from build123d import *

# Parameters (mm, degrees)
F0_R     = 1.5
F0_W     = 3.175
F0_H     = 19.05
F0_W_2   = 10.5
F0_H_2   = 27
F1_DEPTH = 12.7


with BuildPart() as f1:
    # F0 (on Front) → F1 (new body)
    with BuildSketch(Plane.XZ):
        Polygon((-85.725, 161.925), (-161.925, 161.925), (-161.925, 85.725), (-146.685, 72.43161), (-146.685, -72.43161), (-161.925, -85.725), (-161.925, -161.925), (-85.725, -161.925), (-72.43161, -146.685), (72.43161, -146.685), (85.725, -161.925), (161.925, -161.925), (161.925, -85.725), (146.685, -72.43161), (146.685, 72.43161), (161.925, 85.725), (161.925, 161.925), (85.725, 161.925), (72.43161, 146.685), (63.7538, 146.685), (63.7538, -5.715), (-5.2462, -5.715), (-5.2462, 146.685), (-72.43161, 146.685), align=None)
        with Locations((-146.925, -156.925)):
            Circle(F0_R, mode=Mode.SUBTRACT)
        with Locations((-156.925, -146.925)):
            Circle(F0_R, mode=Mode.SUBTRACT)
        with Locations((-153.9875, -123.825)):
            Rectangle(F0_W, F0_H, mode=Mode.SUBTRACT)
        with Locations((-94.9964, -72.225)):
            Circle(F0_R, mode=Mode.SUBTRACT)
        with Locations((-84.9962, -72.225)):
            Rectangle(F0_W_2, F0_H_2, mode=Mode.SUBTRACT)
        with Locations((-74.9964, -72.225)):
            Circle(F0_R, mode=Mode.SUBTRACT)
        with Locations((146.925, -156.925)):
            Circle(F0_R, mode=Mode.SUBTRACT)
        with Locations((156.925, -146.925)):
            Circle(F0_R, mode=Mode.SUBTRACT)
        with Locations((153.9875, -123.825)):
            Rectangle(F0_W, F0_H, mode=Mode.SUBTRACT)
        with Locations((75.0036, -72.225)):
            Circle(F0_R, mode=Mode.SUBTRACT)
        with Locations((85.0038, -72.225)):
            Rectangle(F0_W_2, F0_H_2, mode=Mode.SUBTRACT)
        with Locations((95.0036, -72.225)):
            Circle(F0_R, mode=Mode.SUBTRACT)
        with Locations((-94.9964, 72.225)):
            Circle(F0_R, mode=Mode.SUBTRACT)
        with Locations((-84.9962, 72.225)):
            Rectangle(F0_W_2, F0_H_2, mode=Mode.SUBTRACT)
        with Locations((-74.9964, 72.225)):
            Circle(F0_R, mode=Mode.SUBTRACT)
        with Locations((-153.9875, 123.825)):
            Rectangle(F0_W, F0_H, mode=Mode.SUBTRACT)
        with Locations((-156.925, 146.925)):
            Circle(F0_R, mode=Mode.SUBTRACT)
        with Locations((-146.925, 156.925)):
            Circle(F0_R, mode=Mode.SUBTRACT)
        with Locations((75.0036, 72.225)):
            Circle(F0_R, mode=Mode.SUBTRACT)
        with Locations((85.0038, 72.225)):
            Rectangle(F0_W_2, F0_H_2, mode=Mode.SUBTRACT)
        with Locations((95.0036, 72.225)):
            Circle(F0_R, mode=Mode.SUBTRACT)
        with Locations((153.9875, 123.825)):
            Rectangle(F0_W, F0_H, mode=Mode.SUBTRACT)
        with Locations((156.925, 146.925)):
            Circle(F0_R, mode=Mode.SUBTRACT)
        with Locations((146.925, 156.925)):
            Circle(F0_R, mode=Mode.SUBTRACT)
        Polygon((-146.685, 72.43161), (-161.925, 85.725), (-161.925, -85.725), (-146.685, -72.43161), align=None)
    extrude(amount=F1_DEPTH)


solid = f1.part
Read the model definition and answer for the solid it produces. Units are mm, in the model's axes. A direction names the side the tool comes from. Coordinates: 2 decimals unless noted, no trailing zeros. Loops run counter-clockwise (first coordinate to the right, second up) from the corner with the lowest first, then second, coordinate; pieces in that order, holes last. Notation, with made-up numbers: (-8, 48.25) - (51, 48.25) arc R16 ccw to (51, 70.25) - close; hole circle Ø5 at (26.5, -4.5). An arc over 180 degrees is marked (long way). Answer in a Markdown table with one row per item.
Q1. Straight lines are drawn through the part: line 1 along X through (y, z) = (-8.5, -119) (3 decimals); line 2 along X through (y, z) = (-8.75, -85.5) (3 decimals); line 3 along X through (y, z) = (-3.5, 89) (3 decimals). For each, find the intervals that lie inside material, in ascending order. Write a range as [from, to].
Here are the results:
| item | result |
|---|---|
| line 1 | x = [-161.925, -155.575], [-152.4, 152.4], [155.575, 161.925] |
| line 2 | x = [-161.925, -90.246], [-79.746, 79.754], [90.254, 161.667] |
| line 3 | x = [-161.925, -5.246], [63.754, 161.925] |
Q2. Find section B-B on z = 43. Write down the section's boundary in (x, y) (3 decimals).
Here are the results:
| item | result |
|---|---|
| outline | (-161.925, -12.7) - (-5.246, -12.7) - (-5.246, 0) - (-161.925, 0) - close; (63.754, -12.7) - (146.685, -12.7) - (146.685, 0) - (63.754, 0) - close |
Q3. The mould has two halves that part along X. Classify faces 1 (the flat face through (-161.925, -6, 2)), 2 (the flat face through (79.17, -6.26, 154.41)), 3 (the flat face through (-123, -6, 161.925)), 4 (the flat face through (154.198, -6.261, 78.985)): pulls with the +X half, pulls with the -X half, needs draft (parallel to the pull), parting line crosses it, or undercut.
Here are the results:
| item | result |
|---|---|
| face 1 | pulls with the -X half |
| face 2 | undercut |
| face 3 | needs draft |
| face 4 | pulls with the +X half |
Q4. For faces 5 (the flat face through (154.41, -6.26, -79.17)), 6 (the flat face through (161.925, -6, -124)), 7 (the flat face through (90.254, -6, -72)), 8 (the flat face through (68, -6, 146.685)), 9 (the flat face through (-1, -6, -146.685)), determine the directions among +Z, -Z, +X, -X, +Y, -Y from which every point of the face is accessible in a straight line to the end or side of a thin tool.
Here are the results:
| item | result |
|---|---|
| face 5 | +X, +Y, -Y |
| face 6 | +Z, -Z, +X, +Y, -Y |
| face 7 | +Y, -Y |
| face 8 | +Z, +Y, -Y |
| face 9 | -Z, +Y, -Y |
Q5. Given P1, Ø4, axis at x = -3, y = -9, coming from the -Z side (3 decimals); P2, Ø6, axis at x = -1, z = 112, coming from the -Y side; P3, Ø5, axis at x = -84, y = -6, coming from the -Z side (3 decimals); P4, Ø4, axis at y = -7.5, z = -67.5, coming from the +X side (3 decimals), each flat-ended and moving along its own axis, determine where each tip first touches the part or whether it passes through.
Here are the results:
| item | result |
|---|---|
| P1 | stops at z = -146.685 |
| P2 | passes through |
| P3 | stops at z = -161.925 |
| P4 | stops at x = 146.685 |
Q6. Find section A-A on z = 120. Write down the section's boundary in (x, y) (3 decimals).
Here are the results:
| item | result |
|---|---|
| outline | (-161.925, -12.7) - (-155.575, -12.7) - (-155.575, 0) - (-161.925, 0) - close; (-152.4, -12.7) - (-5.246, -12.7) - (-5.246, 0) - (-152.4, 0) - close; (63.754, -12.7) - (152.4, -12.7) - (152.4, 0) - (63.754, 0) - close; (155.575, -12.7) - (161.925, -12.7) - (161.925, 0) - (155.575, 0) - close |
Q7. Find section D-D on y = -2. Count the separate pieces of the cut face and the enclosed holes in it, plus the area to 3 significant figures.
Here are the results:
| item | result |
|---|---|
| separate pieces | 1 |
| enclosed holes | 24 |
| area | 85,600 mm^2 |
Q8. Find section C-C on x = 56.5. Write down the section's boundary in (y, z) (3 decimals), plus the area to 3 significant figures.
Here are the results:
| item | result |
|---|---|
| outline | (-12.7, -146.685) - (0, -146.685) - (0, -5.715) - (-12.7, -5.715) - close |
| area | 1,790 mm^2 |
